Build history of the part. All positions in model axes, mm. Give positions to 0.01 mm unless a question says otherwise; leave off trailing zeros. Loops run counter-clockwise (first coordinate to the right, second up) from the corner with the lowest first, then second, coordinate; pieces in that order, holes last.
1) Band-saw the part on C-C on z = -3.7. List the corners of the cut face in (x, y).
2) Band-saw the part on D-D on y = 2.2. List the corners of the cut face in (x, z).
3) Flat gauge pin, fed straight in: P1, Ø1, axis at y = 2, z = -3.5, coming from the -X side. Where does the tip first touch, or does it go through?
4) Wall check: line 1 (Y direction, x = 0, z = -2.4); line 2 (Y direction, x = -1.2, z = -0.15); line 3 (X direction, y = -1, z = -3.2). Give the ranges that are in metal, low to high.
5) Band-saw the part on A-A on y = 0. List the corners of the cut face in (x, z), then the cut area to 3 significant figures.
Autodesk Inventor part; units mm, degrees
ref_plane "YZ Plane" through (0, 0, 0) normal (1, 0, 0) x (0, 1, 0)
ref_plane "XZ Plane" through (0, 0, 0) normal (0, 1, 0) x (-1, 0, 0)
ref_plane "XY Plane" through (0, 0, 0) normal (0, 0, 1) x (1, 0, 0)
sketch "Boceto1" plane through (0, 0, 0) normal (0, 0, 1) x (1, 0, 0)
  circle A0 centre (0, 0) radius 1.4 construction
  circle A1 centre (0, 0) radius 1.6
  line L0 (-3, 3) -> (3, 3)
  line L1 (3, 3) -> (3, -3)
  line L2 (3, -3) -> (-3, -3)
  line L3 (-3, -3) -> (-3, 3)
  line L4 (-3, 3) -> (3, -3) construction
  line L5 (3, 3) -> (-3, -3) construction
  point P0 (0, 0)
  point P1 (0, -3)
  dimension "d0" = 0.2
  dimension "d1" = 3
  dimension "d2" = 3
extrude "Extrusión1" add sketch "Boceto1" against normal blind 4
fillet "Empalme1" radius 2 4 edges at (3, -3, -2) (-3, -3, -2) (-3, 3, -2) (3, 3, -2)
properties part number "TapónEje"
Findings below:
1. outline: (-3, -1) arc R2 ccw to (-1, -3) - (1, -3) arc R2 ccw to (3, -1) - (3, 1) arc R2 ccw to (1, 3) - (-1, 3) arc R2 ccw to (-3, 1) - close; hole circle Ø3.2 at (0, 0)
2. outline: (-2.6, -4) - (2.6, -4) - (2.6, 0) - (-2.6, 0) - close
3. P1: stops at x = -2.94
4. line 1: y = -3 to -1.6, 1.6 to 3
4. line 2: y = -2.99 to -1.06, 1.06 to 2.99
4. line 3: x = -3 to -1.25, 1.25 to 3
5. outline: (-3, -4) - (-1.6, -4) - (-1.6, 0) - (-3, 0) - close; (1.6, -4) - (3, -4) - (3, 0) - (1.6, 0) - close
5. area: 11.2 mm2
